Could you check a few things on this model? Use its own coordinates, in mm. Face numbers are marked on the shaded views. A direction names the side the tool comes from. Round coordinates to 2 decimals unless told otherwise and drop trailing zeros. Write each loop counter-clockwise with the first axis right and the second up, starting at its lowest first coordinate (ties: lowest second). Pieces come first, ordered by that corner, then holes. Notation, with made-up numbers: (7, 11.25) -> (51, 11.25) arc R15 ccw to (51, 23.25) -> close; hole circle Ø2 at (68, -16). An arc over 180 degrees is marked (long way). Answer as CSV lines item,"result". Start each with the question number.
Q1. If we mould it in two halves opening along X, with no side actions, what happens to the marked faces 1 and 2? For each: pulls with the +X half, pulls with the -X half, needs draft (parallel to the pull), parting line crosses it, or undercut.
Q2. Will this pin go through, and if not, where does the flat tip stop? pin 1 Ø2 at (x, y) = (-13, -1.5) entering from -Z.
Q3. Imagine slicing it at C-C on y = -4.5. Please give me the cut outline in (x, z), and give its area (3 significant figures).
Q4. For the marked faces 3 and 4, which set-ups out of +Z, -Z, +X, -X, +Y, -Y let a thin tool reach every point of the face, with its end or its side?
Q5. If I drill on line 1 (X direction, y = 0, z = 4.2); line 2 (Y direction, x = 0.5, z = 4.35); line 3 (Z direction, x = -10.5, y = -3.75), over which ranges is the centre line in solid material (lowest first)? Write a range as [from, to].
Q6. Imagine slicing it at D-D on z = 4.2. Please give me the cut outline in (x, y).
Q7. Imagine slicing it at A-A on y = 0. Please give me the cut outline in (x, z), and give its area (3 significant figures).
Q8. Imagine slicing it at B-B on x = 0. Please give me the cut outline in (y, z), and give its area (3 significant figures).
Solid Edge part; units mm, degrees
sketch "Sketch1" plane through (0, 0, 0) normal (0, -1, 0) x (1, 0, 0)
  line L0 (6.5374, 3.6848) -> (-43.4626, 3.6848)
  line L1 (6.5374, 4.4848) -> (6.5374, 3.6848)
  line L2 (6.5374, 4.4848) -> (-43.4626, 4.4848)
  line L3 (-43.4626, 3.6848) -> (-43.4626, 4.4848)
  dimension "D1" = 6.5374
extrude "Protrusion1" add sketch "Sketch1" along normal mid plane 10
sketch "Sketch2" plane through (-22.7754, 0, 5) normal (0, 0, 1) x (0, -1, 0)
  circle A0 centre (0, 23.3128) radius 2.2
extrude "Cutout1" cut sketch "Sketch2" along normal through all and the other way through all
sketch "Sketch3" plane through (-18.4626, 0, 4.4848) normal (0, 0, 1) x (1, 0, 0)
  line L0 (9, 5) -> (9, -5)
  line L1 (9, -5) -> (2, -5)
  line L2 (2, -5) -> (2, 5)
  line L3 (2, 5) -> (9, 5)
extrude "ExtrudedCutout_3" cut sketch "Sketch3" against normal blind 0.1
sketch "Sketch4" plane through (-18.4626, 0, 3.6848) normal (0, 0, -1) x (1, 0, 0)
  line L0 (2, 5) -> (2, -5)
  line L1 (9, -5) -> (2, -5)
  line L2 (9, -5) -> (9, 5)
  line L3 (2, 5) -> (9, 5)
extrude "ExtrudedCutout_4" cut sketch "Sketch4" against normal blind 0.1
properties material "Steel"
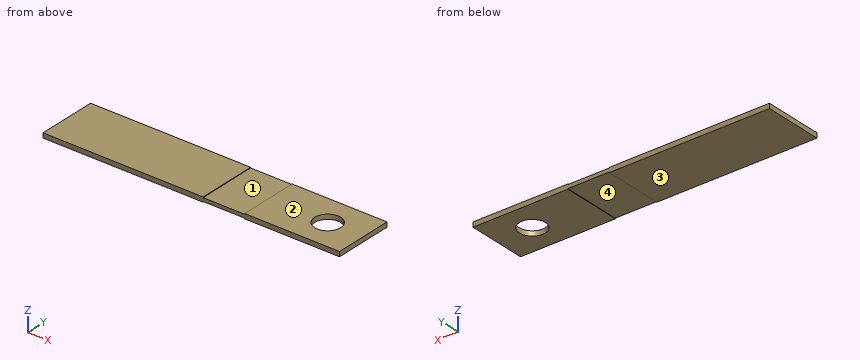
Checks:
1,face 1,"undercut"
1,face 2,"needs draft"
2,pin 1,"z = 3.78"
3,outline,"(-43.46, 3.68) -> (-16.46, 3.68) -> (-16.46, 3.78) -> (-9.46, 3.78) -> (-9.46, 3.68) -> (6.54, 3.68) -> (6.54, 4.48) -> (-9.46, 4.48) -> (-9.46, 4.38) -> (-16.46, 4.38) -> (-16.46, 4.48) -> (-43.46, 4.48) -> close"
3,area,"38.6 mm^2"
4,face 3,"-Z, +X, -X, +Y, -Y"
4,face 4,"-Z, +Y, -Y"
5,line 1,"[-43.46, -1.66], [2.74, 6.54]"
5,line 2,"[-5, -2.2], [2.2, 5]"
5,line 3,"[3.78, 4.38]"
6,outline,"(-43.46, -5) -> (6.54, -5) -> (6.54, 5) -> (-43.46, 5) -> close; hole circle Ø4.4 at (0.54, 0)"
7,outline,"(-43.46, 3.68) -> (-16.46, 3.68) -> (-16.46, 3.78) -> (-9.46, 3.78) -> (-9.46, 3.68) -> (-1.66, 3.68) -> (-1.66, 4.48) -> (-9.46, 4.48) -> (-9.46, 4.38) -> (-16.46, 4.38) -> (-16.46, 4.48) -> (-43.46, 4.48) -> close; (2.74, 3.68) -> (6.54, 3.68) -> (6.54, 4.48) -> (2.74, 4.48) -> close"
7,area,"35.1 mm^2"
8,outline,"(-5, 3.68) -> (-2.13, 3.68) -> (-2.13, 4.48) -> (-5, 4.48) -> close; (2.13, 3.68) -> (5, 3.68) -> (5, 4.48) -> (2.13, 4.48) -> close"
8,area,"4.59 mm^2"
